For this review, use the dimensioned drawing (mm, ordinates from the lowest corner) and the shaded views. Round coordinates to 2 decimals unless told otherwise and drop trailing zeros. Write each loop counter-clockwise with the first axis right and the second up, starting at its lowest first coordinate (ties: lowest second). Pieces come first, ordered by that corner, then holes. Notation, with made-up numbers: M 5,-27.75 L 60,-27.75 A20 ccw 60,-16.75 Z; hole C 38,29.25 d4. An arc over 180 degrees is marked long. Write each question's results on one line, items separated by ' | '. Start each with the question number.
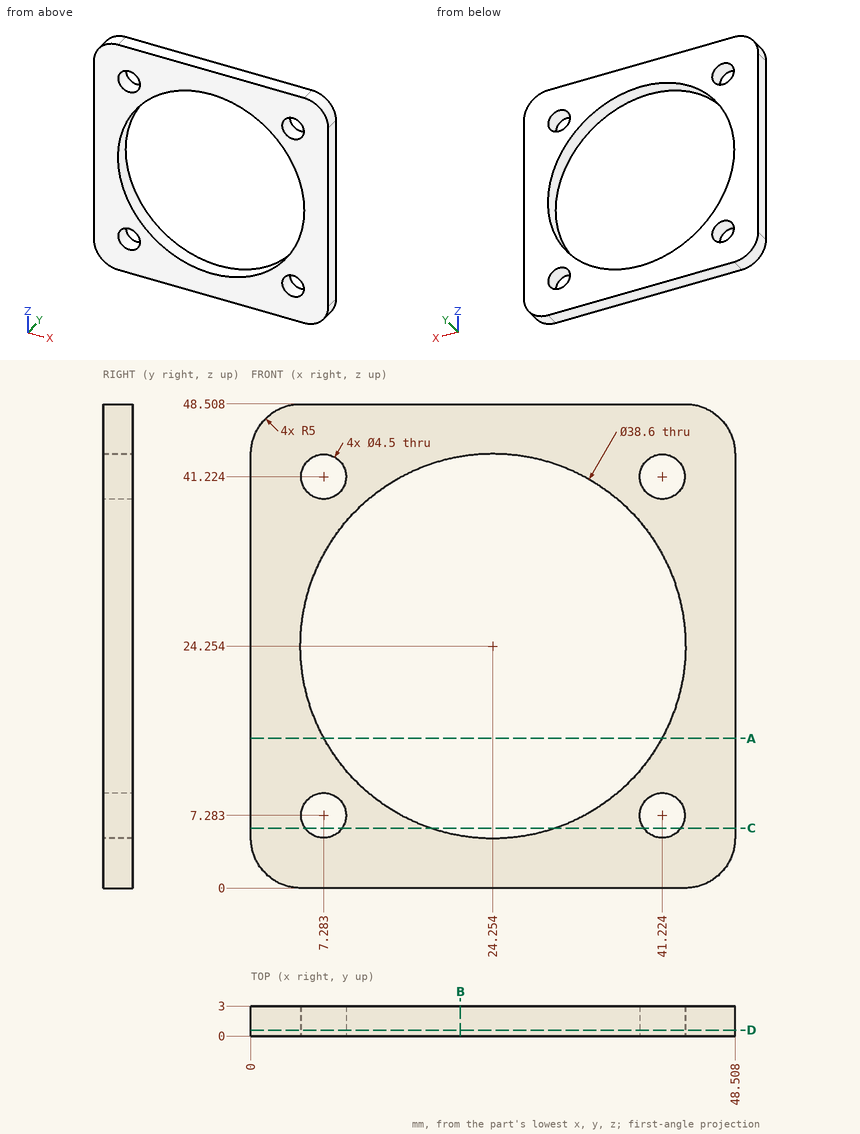
Item 1: For probe 1 along Z at (x, y) = (22.5, 0.55) (1 decimal); probe 2 along Z at (x, y) = (42, 0.75) (1 decimal); probe 3 along Z at (x, y) = (40, 1.2) (1 decimal), list the stretches that pass through material, from the lowest coordinate up.
Item 2: We need section B-B on x = 21. State the section outline as (y, z) points.
Item 3: We need section C-C on z = 6. State the section outline as (x, y) points (1 decimal).
Item 4: We need section A-A on z = 15. State the section outline as (x, y) points.
Item 5: We need section D-D on y = 0.6. State how many separate pieces and enclosed holes the cut face has, then the cut area to 3 significant figures.
Numbers:
1) probe 1: z = 0 to 5, 43.5 to 48.5 | probe 2: z = 0 to 5.2, 9.4 to 16.7, 31.8 to 39.1, 43.3 to 48.5 | probe 3: z = 0 to 5.4, 9.2 to 13.1, 35.4 to 39.3, 43.1 to 48.5
2) outline: M 0,0 L 3,0 L 3,5.23 L 0,5.23 Z; M 0,43.28 L 3,43.28 L 3,48.51 L 0,48.51 Z
3) outline: M 0,0 L 5.4,0 L 5.4,3 L 0,3 Z; M 9.1,0 L 18,0 L 18,3 L 9.1,3 Z; M 30.5,0 L 39.4,0 L 39.4,3 L 30.5,3 Z; M 43.1,0 L 48.5,0 L 48.5,3 L 43.1,3 Z
4) outline: M 0,0 L 7.32,0 L 7.32,3 L 0,3 Z; M 41.19,0 L 48.51,0 L 48.51,3 L 41.19,3 Z
5) separate pieces: 1 | enclosed holes: 5 | area: 1,100 mm^2
